Geometry check sheet. Reference: the model listing, model coordinates, mm. A direction names the side the tool comes from. Coordinates: 2 decimals unless noted, no trailing zeros. Write each loop counter-clockwise with the first axis right and the second up, starting at its lowest first coordinate (ties: lowest second). Pieces come first, ordered by that corner, then holes. Notation, with made-up numbers: (70, 56) -> (115, 56) arc R27 cw to (115, 72) -> close; hole circle Ø2 at (55.25, 69.5). An arc over 180 degrees is marked (long way). Use a Markdown table: item, result.
```python
from build123d import *

# Parameters (mm, degrees)
SKETCH1_R      = 72.3
EXTRUDE1_DEPTH = 2.54
SKETCH2_R      = 6.35
EXTRUDE2_DEPTH = 103.279184588
SKETCH3_R      = 33.25
EXTRUDE3_DEPTH = 103.279184588
EXTRUDE4_DEPTH = 2.54
FILLET1_R      = 2.54


with BuildPart() as part:
    # Sketch1 → Extrude1 (new body)
    with BuildSketch(Plane(origin=(0, 0, 0), x_dir=(1, 0, 0), z_dir=(0, 1, 0))):
        with Locations(Location((0, 0, 0), (0, 0, 270))):
            Circle(SKETCH1_R)
    extrude(amount=EXTRUDE1_DEPTH)

    # Sketch2 → Extrude2 (cut, through all)
    with BuildSketch(Plane.XZ):
        with Locations(Location((-58.42, 0, 0), (0, 0, 270))):
            Circle(SKETCH2_R)
        with Locations(Location((58.42, 0, 0), (0, 0, 90))):
            Circle(SKETCH2_R)
        with Locations(Location((0, 58.42, 0), (0, 0, 270))):
            Circle(SKETCH2_R)
    extrude(amount=-EXTRUDE2_DEPTH, mode=Mode.SUBTRACT)

    # Sketch3 → Extrude3 (cut, through all)
    with BuildSketch(Plane.XZ):
        with Locations(Location((0, 0, 0), (0, 0, 270))):
            Circle(SKETCH3_R)
    extrude(amount=-EXTRUDE3_DEPTH, mode=Mode.SUBTRACT)

    # Sketch4 → Extrude4 (cut)
    with BuildSketch(Plane.XZ):
        with BuildLine():
            Line((-42.239772226, -17.496286528), (-196.027114776, -81.197089533))
            Line((-196.027114776, -81.197089533), (196.027114776, -81.197089533))
            Line((196.027114776, -81.197089533), (42.239772226, -17.496286528))
            ThreePointArc((42.239772226, -17.496286528), (0, -45.72), (-42.239772226, -17.496286528))
        make_face()
        with BuildLine():
            Line((-42.239772226, 17.496286528), (-90.262778901, 37.388067198))
            Line((-90.262778901, 37.388067198), (-35.092483391, 84.720749339))
            Line((-35.092483391, 84.720749339), (-17.496286528, 42.239772226))
            ThreePointArc((-17.496286528, 42.239772226), (-32.328922036, 32.328922036), (-42.239772226, 17.496286528))
        make_face()
        with BuildLine():
            Line((42.239772226, 17.496286528), (90.262778901, 37.388067198))
            Line((90.262778901, 37.388067198), (35.092483391, 84.720749339))
            Line((35.092483391, 84.720749339), (17.496286528, 42.239772226))
            ThreePointArc((17.496286528, 42.239772226), (32.328922036, 32.328922036), (42.239772226, 17.496286528))
        make_face()
    extrude(amount=-EXTRUDE4_DEPTH, mode=Mode.SUBTRACT)

    # Fillet1
    fillet1_edges = [part.edges().sort_by_distance(p)[0] for p in [
        (66.796490201, 1.27, -27.66801216),
        (42.239772226, 1.27, -17.496286528),
        (-66.796490201, 1.27, -27.66801216),
        (-42.239772226, 1.27, -17.496286528),
        (-66.796490201, 1.27, 27.66801216),
        (-42.239772226, 1.27, 17.496286528),
        (-27.66801216, 1.27, 66.796490201),
        (-17.496286528, 1.27, 42.239772226),
        (27.66801216, 1.27, 66.796490201),
        (17.496286528, 1.27, 42.239772226),
        (66.796490201, 1.27, 27.66801216),
        (42.239772226, 1.27, 17.496286528),
    ]]
    fillet(fillet1_edges, radius=FILLET1_R)


solid = part.part
```
Item 1: Section check A-A on x = 0. Record the boundary of the cut face in (y, z).
Answer block:
| item | result |
|---|---|
| outline | (0, -45.72) -> (2.54, -45.72) -> (2.54, -33.25) -> (0, -33.25) -> close; (0, 33.25) -> (2.54, 33.25) -> (2.54, 52.07) -> (0, 52.07) -> close; (0, 64.77) -> (2.54, 64.77) -> (2.54, 72.3) -> (0, 72.3) -> close |
Item 2: Tool access check on faces 4 (the cylindrical face through (32.175, 1.252, 32.482)), 5 (the flat face through (54.327, 1.252, 22.503)), 6 (the flat face through (22.62, 1.25, 54.61)), 7 (the flat face through (-54.327, 1.252, -22.503)), 8 (the flat face through (-22.62, 1.25, 54.61)). Record the directions out of +Z, -Z, +X, -X, +Y, -Y that give a thin tool (end or side, any length) a straight path to the whole face; none if there is none.
Answer block:
| item | result |
|---|---|
| face 4 | +Y, -Y |
| face 5 | +Z, +Y, -Y |
| face 6 | +X, +Y, -Y |
| face 7 | -Z, +Y, -Y |
| face 8 | -X, +Y, -Y |
Item 3: Section check C-C on y = 0.4. Record the boundary of the cut face in (x, z).
Answer block:
| item | result |
|---|---|
| outline | (-67.76, -25.22) arc R2.54 ccw to (-64.41, -26.68) -> (-44.52, -18.44) arc R2.54 cw to (-41.26, -19.7) arc R45.72 ccw to (41.26, -19.7) arc R2.54 cw to (44.52, -18.44) -> (64.41, -26.68) arc R2.54 ccw to (67.76, -25.22) arc R72.3 ccw to (67.76, 25.22) arc R2.54 ccw to (64.41, 26.68) -> (44.52, 18.44) arc R2.54 cw to (41.26, 19.7) arc R45.72 ccw to (19.7, 41.26) arc R2.54 cw to (18.44, 44.52) -> (26.68, 64.41) arc R2.54 ccw to (25.22, 67.76) arc R72.3 ccw to (-25.22, 67.76) arc R2.54 ccw to (-26.68, 64.41) -> (-18.44, 44.52) arc R2.54 cw to (-19.7, 41.26) arc R45.72 ccw to (-41.26, 19.7) arc R2.54 cw to (-44.52, 18.44) -> (-64.41, 26.68) arc R2.54 ccw to (-67.76, 25.22) arc R72.3 ccw to start; hole circle Ø12.7 at (-58.42, 0); hole circle Ø66.5 at (0, 0); hole circle Ø12.7 at (0, 58.42); hole circle Ø12.7 at (58.42, 0) |
Item 4: Section check B-B on z = 0. Record the boundary of the cut face in (x, y).
Answer block:
| item | result |
|---|---|
| outline | (-72.3, 0) -> (-64.77, 0) -> (-64.77, 2.54) -> (-72.3, 2.54) -> close; (-52.07, 0) -> (-33.25, 0) -> (-33.25, 2.54) -> (-52.07, 2.54) -> close; (33.25, 0) -> (52.07, 0) -> (52.07, 2.54) -> (33.25, 2.54) -> close; (64.77, 0) -> (72.3, 0) -> (72.3, 2.54) -> (64.77, 2.54) -> close |
Item 5: Section check D-D on x = -15. Record the boundary of the cut face in (y, z), then the cut area to 3 significant figures.
Answer block:
| item | result |
|---|---|
| outline | (0, -43.19) -> (2.54, -43.19) -> (2.54, -29.67) -> (0, -29.67) -> close; (0, 29.67) -> (2.54, 29.67) -> (2.54, 70.73) -> (0, 70.73) -> close |
| area | 139 mm^2 |
Item 6: Mould release check, pull along Z, two halves, no side actions. Record for faces 1 (the flat face through (54.61, 1.25, -22.62)), 2 (the cylindrical face through (72.3, 1.3, 0.4)), 3 (the cylindrical face through (64.62, 1.25, -1.38)): +Z half, -Z half, draft (parallel to the pull), parting line (faces both ways), or undercut.
Answer block:
| item | result |
|---|---|
| face 1 | -Z half |
| face 2 | parting line |
| face 3 | undercut |
Item 7: Thickness scan on L1, parallel to X at y = 0.8, z = 0; L2, parallel to X at y = 0.65, z = 0.5; L3, parallel to X at y = 0.8, z = -37. Record the ranges inside material, lowest first. Write a range as [from, to].
Answer block:
| item | result |
|---|---|
| L1 | x = [-72.3, -64.77], [-52.07, -33.25], [33.25, 52.07], [64.77, 72.3] |
| L2 | x = [-72.3, -64.75], [-52.09, -33.25], [33.25, 52.09], [64.75, 72.3] |
| L3 | x = [-26.86, 26.86] |
